from build123d import *

# Parameters (mm, degrees)
SM_BASE_FLANGE_1_DEPTH = 56.4
FILLET_1_R             = 3
SKETCH_6_R             = 20
SKETCH_6_R_2           = 2.55
CUT_EXTRUDE_1_DEPTH    = 148.256239257


# Sheet-metal steps are written as plain solids
with BuildPart() as part:
    # Sketch 1 → Базовая кромка1 (new body)
    with BuildSketch(Plane.XY):
        with BuildLine():
            Line((0, 0), (0, -100.2))
            ThreePointArc((0, -100.2), (0.878679656, -102.321320344), (3, -103.2))
            Line((3, -103.2), (85, -103.2))
            Line((85, -103.2), (85, -106.2))
            Line((85, -106.2), (3, -106.2))
            ThreePointArc((3, -106.2), (-1.242640687, -104.442640687), (-3, -100.2))
            Line((-3, -100.2), (-3, 0))
            Line((-3, 0), (0, 0))
        make_face()
    extrude(amount=SM_BASE_FLANGE_1_DEPTH)

    # Скругление1
    fillet_1_edges = [part.edges().sort_by_distance(p)[0] for p in [
        (-1.5, 0, 56.4),
        (85, -104.7, 56.4),
        (-1.5, 0, 0),
        (85, -104.7, 0),
    ]]
    fillet(fillet_1_edges, radius=FILLET_1_R)

    # Эскиз6 → Вырез-Вытянуть1 (cut, through all)
    with BuildSketch(Plane(origin=(0, 0, 0), x_dir=(0, 0, -1), z_dir=(1, 0, 0))):
        with Locations(Location((-28.2, -28.2, 0), (0, 0, 90))):
            Circle(SKETCH_6_R)
        with Locations(Location((-51.77, -4.63, 0), (0, 0, 90))):
            Circle(SKETCH_6_R_2)
        with Locations(Location((-4.63, -4.63, 0), (0, 0, 90))):
            Circle(SKETCH_6_R_2)
        with Locations(Location((-4.63, -51.77, 0), (0, 0, 90))):
            Circle(SKETCH_6_R_2)
        with Locations(Location((-51.77, -51.77, 0), (0, 0, 90))):
            Circle(SKETCH_6_R_2)
    extrude(amount=-CUT_EXTRUDE_1_DEPTH, mode=Mode.SUBTRACT)


solid = part.part
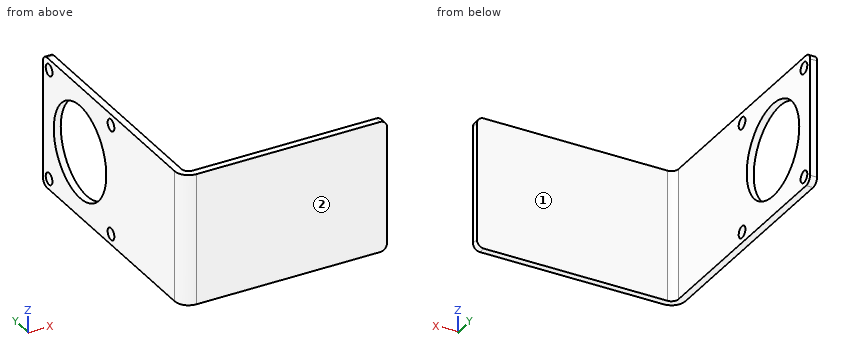
Part model, mm, in its own coordinate system. Face numbers are marked on the shaded views. A direction names the side the tool comes from. Coordinates: 2 decimals unless noted, no trailing zeros. Loops run counter-clockwise (first coordinate to the right, second up) from the corner with the lowest first, then second, coordinate; pieces in that order, holes last. Notation, with made-up numbers: (7, 23.25) -> (25, 23.25) arc R16 ccw to (25, 37.25) -> close; hole circle Ø9 at (-17.75, -27). An arc over 180 degrees is marked (long way). Use a Markdown table: item, result. Add a question column.
Item 1: Band-saw the part on B-B on z = 28.2. Write the cut outline in (x, y), plus the area to 3 significant figures.
Item 2: Band-saw the part on C-C on z = 51.77. Write the cut outline in (x, y).
Item 3: Which spindle directions (+Z, -Z, +X, -X, +Y, -Y) get a long thin tool onto all of the face, cutting with end or side? Do the marked faces 1 and 2. Say none if no direction does.
Item 4: Band-saw the part on A-A on y = -4.63. Write the cut outline in (x, z), plus the area to 3 significant figures.
Item 5: Band-saw the part on D-D on y = -28.2. Write the cut outline in (x, z), plus the area to 3 significant figures.
Item 6: Probe probe 1 along Z at (x, y) = (-1.55, -51.77); probe 2 along Z at (x, y) = (-2, -4); probe 3 along X at (y, z) = (-67.5, 45). List the from-to ranges inside material, lowest first.
Item 7: Flat gauge pins, fed straight in: P1, Ø1.5, axis at x = 46.5, z = 39, coming from the +Y side; P2, Ø5, axis at y = -76.5, z = 39, coming from the +X side. Where does each tip first touch, or does it go through?
Geometry says:
| question | item | result |
|---|---|---|
| 1 | outline | (-3, -100.2) arc R6 ccw to (3, -106.2) -> (85, -106.2) -> (85, -103.2) -> (3, -103.2) arc R3 cw to (0, -100.2) -> (0, -48.2) -> (-3, -48.2) -> close; (-3, -8.2) -> (0, -8.2) -> (0, 0) -> (-3, 0) -> close |
| 1 | area | 448 mm² |
| 2 | outline | (-3, -100.2) arc R6 ccw to (3, -106.2) -> (85, -106.2) -> (85, -103.2) -> (3, -103.2) arc R3 cw to (0, -100.2) -> (0, -54.32) -> (-3, -54.32) -> close; (-3, -49.22) -> (0, -49.22) -> (0, -7.18) -> (-3, -7.18) -> close; (-3, -2.08) -> (0, -2.08) -> (0, 0) -> (-3, 0) -> close |
| 3 | face 1 | +Z, -Z, +X, +Y |
| 3 | face 2 | +Z, -Z, +X, -X, -Y |
| 4 | outline | (-3, 0) -> (0, 0) -> (0, 2.08) -> (-3, 2.08) -> close; (-3, 7.18) -> (0, 7.18) -> (0, 49.22) -> (-3, 49.22) -> close; (-3, 54.32) -> (0, 54.32) -> (0, 56.4) -> (-3, 56.4) -> close |
| 4 | area | 139 mm² |
| 5 | outline | (-3, 0) -> (0, 0) -> (0, 8.2) -> (-3, 8.2) -> close; (-3, 48.2) -> (0, 48.2) -> (0, 56.4) -> (-3, 56.4) -> close |
| 5 | area | 49.2 mm² |
| 6 | probe 1 | 0 to 2.08, 7.18 to 49.22, 54.32 to 56.4 |
| 6 | probe 2 | 0 to 2.16, 7.1 to 49.3, 54.24 to 56.4 |
| 6 | probe 3 | -3 to 0 |
| 7 | P1 | y = -103.2 |
| 7 | P2 | x = 0 |
